```python
from build123d import *

# Parameters (mm, degrees)
SKETCH1_W               = 12.7
SKETCH1_H               = 133.35
BOSS_EXTRUDE1_DEPTH     = 4.445
CUT_EXTRUDE1_DEPTH      = 68.564119361
CUT_EXTRUDE1_DEPTH_BACK = 68.564119361
SKETCH2_R               = 1.2
SKETCH3_R               = 1.2
CUT_EXTRUDE2_DEPTH      = 12
SKETCH4_W               = 5.65
SKETCH4_H               = 5
CUT_EXTRUDE3_DEPTH      = 69.019141791
SKETCH5_R               = 1.054294776
CUT_EXTRUDE4_DEPTH      = 68.564119361


with BuildPart() as part:
    # Sketch1 → Boss-Extrude1 (new, symmetric)
    with BuildSketch(Plane(origin=(0, 0, 0), x_dir=(1, 0, 0), z_dir=(0, 1, 0))):
        Rectangle(SKETCH1_W, SKETCH1_H)
    extrude(amount=BOSS_EXTRUDE1_DEPTH, both=True)

    # Sketch2 → Cut-Extrude1 (cut, two sides: drawn at the far end of the back side and taken through both)
    with BuildSketch(Plane.XZ.offset(4.445).offset(-CUT_EXTRUDE1_DEPTH_BACK)):
        with Locations(Location((0, 57.15, 0), (0, 0, 270))):
            Circle(SKETCH2_R)
        with Locations(Location((0, 63.5, 0), (0, 0, 270))):
            Circle(SKETCH2_R)
    extrude(amount=CUT_EXTRUDE1_DEPTH + CUT_EXTRUDE1_DEPTH_BACK, mode=Mode.SUBTRACT)

    # Sketch3 → Cut-Extrude2 (cut)
    with BuildSketch(Plane(origin=(0, 0, -66.675), x_dir=(-1, 0, 0), z_dir=(0, 0, -1))):
        Circle(SKETCH3_R)
    extrude(amount=-CUT_EXTRUDE2_DEPTH, mode=Mode.SUBTRACT)

    # Sketch4 → Cut-Extrude3 (cut, through all)
    with BuildSketch(Plane(origin=(6.35, 0, 0), x_dir=(0, 0, -1), z_dir=(1, 0, 0))):
        with Locations((57.5, 0)):
            Rectangle(SKETCH4_W, SKETCH4_H)
    extrude(amount=-CUT_EXTRUDE3_DEPTH, mode=Mode.SUBTRACT)

    # Sketch5 → Cut-Extrude4 (cut, through all)
    with BuildSketch(Plane.XZ.offset(4.445)):
        with Locations(Location((3.015690418, -48.331496192, 0), (0, 0, 270))):
            Circle(SKETCH5_R)
        with Locations(Location((3.015690418, -22.739006486, 0), (0, 0, 270))):
            Circle(SKETCH5_R)
        with Locations(Location((3.015690418, 2.918503808, 0), (0, 0, 270))):
            Circle(SKETCH5_R)
        with Locations(Location((3.015690418, 28.510993514, 0), (0, 0, 270))):
            Circle(SKETCH5_R)
    extrude(amount=-CUT_EXTRUDE4_DEPTH, mode=Mode.SUBTRACT)


solid = part.part
```
CAD build for the part. Positions are in the model's coordinates, mm. A direction names the side the tool comes from. Give positions to 0.01 mm unless a question says otherwise; leave off trailing zeros. Loops run counter-clockwise (first coordinate to the right, second up) from the corner with the lowest first, then second, coordinate; pieces in that order, holes last. Notation, with made-up numbers: (54.25, 86) -> (86.25, 86) arc R22 cw to (86.25, 93) -> close; hole circle Ø8 at (67, 45.25). An arc over 180 degrees is marked (long way). Use a Markdown table: item, result.
1. Slice it at B-B (y = 0). Give the number of separate pieces and of enclosed holes in the cut face, plus the area to 3 significant figures.
Check result:
| item | result |
|---|---|
| separate pieces | 3 |
| enclosed holes | 6 |
| area | 1,580 mm^2 |
2. Wall check: L1, parallel to X at y = 0.25, z = 63.5; L2, parallel to Y at x = 3.75, z = -56 (3 decimals); L3, parallel to Z at x = -3.75, y = 0.5 (3 decimals). Give the ranges that are in metal, low to high. Write a range as [from, to].
Check result:
| item | result |
|---|---|
| L1 | x = [-6.35, -1.2], [1.2, 6.35] |
| L2 | y = [-4.445, -2.5], [2.5, 4.445] |
| L3 | z = [-66.675, -60.325], [-54.675, 66.675] |
3. Slice it at A-A (z = 63.5). List the corners of the cut face in (x, y) (3 decimals), plus the area to 3 significant figures.
Check result:
| item | result |
|---|---|
| outline | (-6.35, -4.445) -> (-1.2, -4.445) -> (-1.2, 4.445) -> (-6.35, 4.445) -> close; (1.2, -4.445) -> (6.35, -4.445) -> (6.35, 4.445) -> (1.2, 4.445) -> close |
| area | 91.6 mm^2 |
4. Mould opens along Z. For faces 3 (the flat face through (-2, 0, -66.675)), 4 (the cylindrical face through (-0.65, 1.01, -63.54)), 5 (the cylindrical face through (2.61, -0.06, -23.71)), 6 (the flat face through (0, 0, 66.675)) say: pulls with the +Z half, pulls with the -Z half, needs draft (parallel to the pull), parting line crosses it, or undercut.
Check result:
| item | result |
|---|---|
| face 3 | pulls with the -Z half |
| face 4 | needs draft |
| face 5 | undercut |
| face 6 | pulls with the +Z half |
5. Slice it at C-C (x = -3). List the corners of the cut face in (y, z) (3 decimals), plus the area to 3 significant figures.
Check result:
| item | result |
|---|---|
| outline | (-4.445, -66.675) -> (4.445, -66.675) -> (4.445, 66.675) -> (-4.445, 66.675) -> close; hole (-2.5, -60.325) -> (2.5, -60.325) -> (2.5, -54.675) -> (-2.5, -54.675) -> close |
| area | 1,160 mm^2 |
6. Which spindle directions (+Z, -Z, +X, -X, +Y, -Y) get a long thin tool onto all of the face, cutting with end or side? Do faces 1 (the flat face through (0, -2.5, -57)), 2 (the cylindrical face through (3.06, -0.06, -47.28)). Say none if no direction does.
Check result:
| item | result |
|---|---|
| face 1 | +X, -X |
| face 2 | +Y, -Y |
